For this review, use the dimensioned drawing (mm, ordinates from the lowest corner) and the shaded views. Coordinates: 2 decimals unless noted, no trailing zeros. Loops run counter-clockwise (first coordinate to the right, second up) from the corner with the lowest first, then second, coordinate; pieces in that order, holes last. Notation, with made-up numbers: (-10, -15) - (5, -15) arc R13 cw to (5, -9) - close; hole circle Ø2 at (31, 11.5). An arc over 180 degrees is marked (long way). Answer in a Markdown table with one row per item. Add a question column.
(1) We need section B-B, the plane x = 0.9. Write out the cut boundary in (y, z).
(2) The part is to be moulded in two halves that separate along Z. For the marked faces 1, 2 and 3, say which applies: released by +Z, released by -Z, zero draft, split by the parting line, or undercut.
(3) Clearance check with a flat-ended pin moving along its axis: pin 1 (3 mm diameter, centred on y = 4.04, z = 3.5, fed in from -X). State where the tip first meets the part, or that it passes through.
(4) To check wall thickness, follow L1, parallel to Z at x = 2.85, y = 4; L2, parallel to Z at x = 2.5, y = 4.75; L3, parallel to Y at x = 2.4, z = 4.5 (1 decimal). State the ranges of each line that lie inside material, in increasing order. Write a range as [from, to].
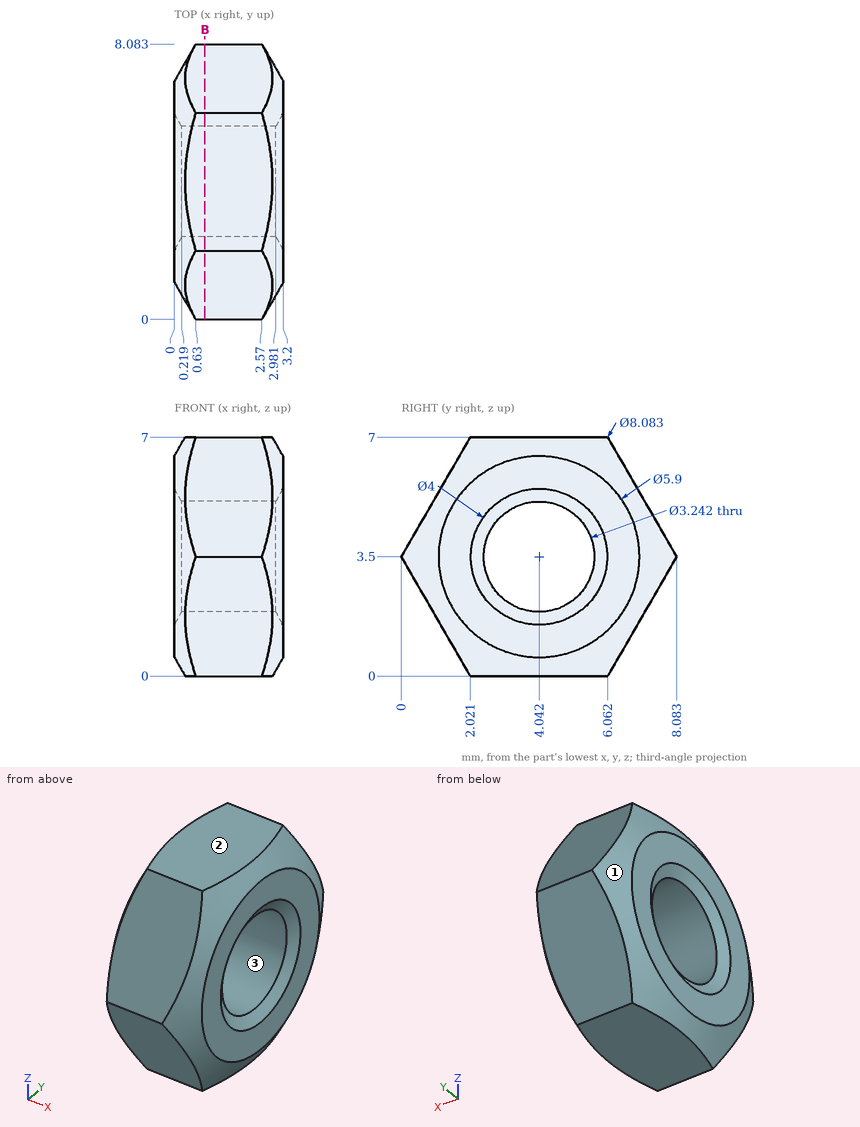
Responses:
| question | item | result |
|---|---|---|
| 1 | outline | (0, 3.5) - (2.02, 0) - (6.06, 0) - (8.08, 3.5) - (6.06, 7) - (2.02, 7) - close; hole circle Ø3.24 at (4.04, 3.5) |
| 2 | face 1 | split by the parting line |
| 2 | face 2 | released by +Z |
| 2 | face 3 | undercut |
| 3 | pin 1 | passes through |
| 4 | L1 | z = [0, 1.88], [5.12, 7] |
| 4 | L2 | z = [0, 2.04], [4.96, 7] |
| 4 | L3 | y = [0.6, 2.8], [5.3, 7.5] |
